Answer from the drawing. Dimensions are ordinates in mm from the lowest x, y and z of the part. A direction names the side the tool comes from. Round coordinates to 2 decimals unless told otherwise and drop trailing zeros. Write each loop counter-clockwise with the first axis right and the second up, starting at its lowest first coordinate (ties: lowest second). Pieces come first, ordered by that corner, then holes. Notation, with made-up numbers: (67, 76) - (89, 76) arc R16 cw to (89, 88) - close; hole circle Ø6 at (-36.5, 38). An arc over 180 degrees is marked (long way). Answer as a JSON object with one key per item and string values.
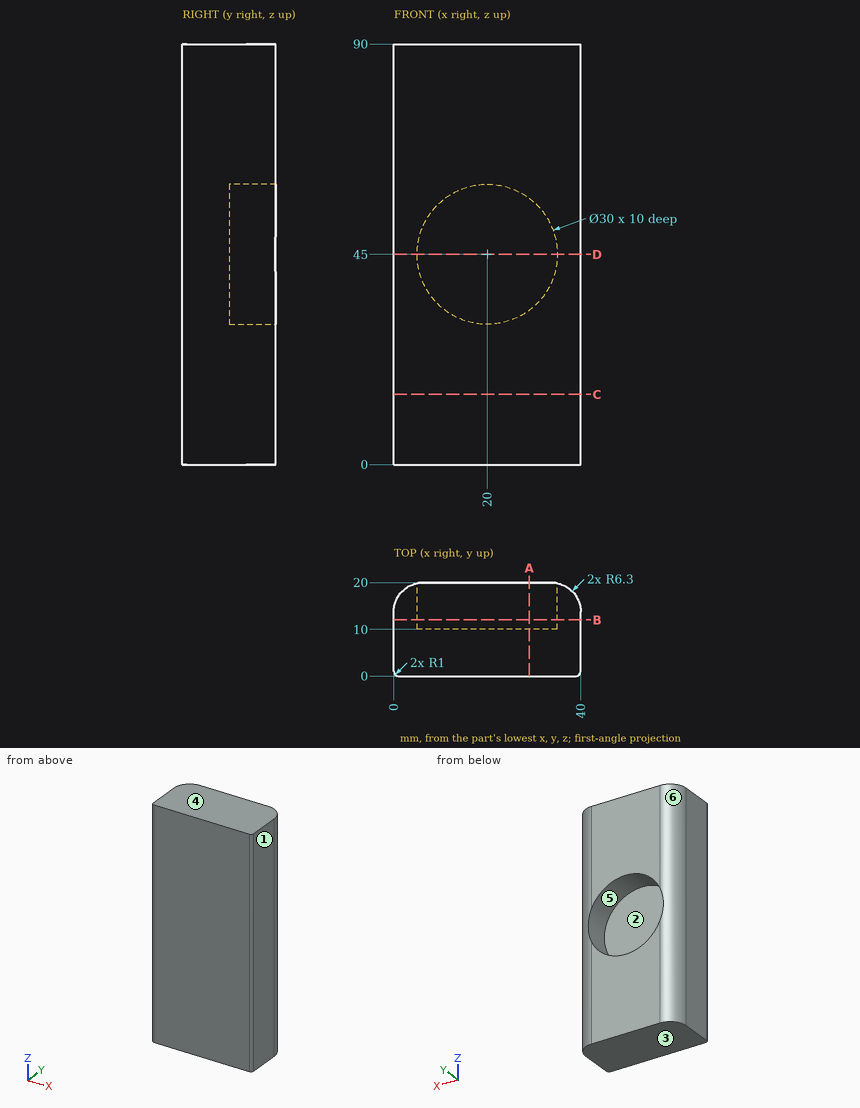
Item 1: Consider line 1 along X through (y, z) = (13.5, 45); line 2 along Y through (x, z) = (23, 37.5); line 3 along X through (y, z) = (15, 51). Determine where each line is inside the solid, lowest interval first.
Results found:
{"line 1": "0 to 5, 35 to 40", "line 2": "0 to 10", "line 3": "0.14 to 6.25, 33.75 to 39.86"}
Item 2: A cutting plane is placed at B-B (y = 12). Write down the section's boundary in (x, z).
Results found:
{"outline": "(0, 0) - (40, 0) - (40, 90) - (0, 90) - close; hole circle Ø30 at (20, 45)"}
Item 3: A cutting plane is placed at A-A (x = 29). Write down the section's boundary in (y, z), and give its area (3 significant figures).
Results found:
{"outline": "(0, 0) - (20, 0) - (20, 33) - (10, 33) - (10, 57) - (20, 57) - (20, 90) - (0, 90) - close", "area": "1,560 mm²"}
Item 4: This flat-tipped pin is pushed along its axis until it touches: P1, Ø15, axis at x = 15, z = 44.5, coming from the +Y side. Where does it stop, or does it pass through?
Results found:
{"P1": "y = 10"}
Item 5: Determine the mould class of the marked faces 3, 4, 5 and 6 for opening direction Z: pulls with the +Z half, pulls with the -Z half, needs draft (parallel to the pull), parting line crosses it, or undercut.
Results found:
{"face 3": "pulls with the -Z half", "face 4": "pulls with the +Z half", "face 5": "undercut", "face 6": "needs draft"}
Item 6: A cutting plane is placed at D-D (z = 45). Write down the section's boundary in (x, y), and give its area (3 significant figures).
Results found:
{"outline": "(0, 1) arc R1 ccw to (1, 0) - (39, 0) arc R1 ccw to (40, 1) - (40, 13.7) arc R6.3 ccw to (35, 19.86) - (35, 10) - (5, 10) - (5, 19.86) arc R6.3 ccw to (0, 13.7) - close", "area": "483 mm²"}
Item 7: For the marked faces 1 and 2, determine the directions among +Z, -Z, +X, -X, +Y, -Y from which every point of the face is accessible in a straight line to the end or side of a thin tool.
Results found:
{"face 1": "+Z, -Z, +X, +Y, -Y", "face 2": "+Y"}
Item 8: A cutting plane is placed at C-C (z = 15). Write down the section's boundary in (x, y), and give its area (3 significant figures).
Results found:
{"outline": "(0, 1) arc R1 ccw to (1, 0) - (39, 0) arc R1 ccw to (40, 1) - (40, 13.7) arc R6.3 ccw to (33.7, 20) - (6.3, 20) arc R6.3 ccw to (0, 13.7) - close", "area": "783 mm²"}
